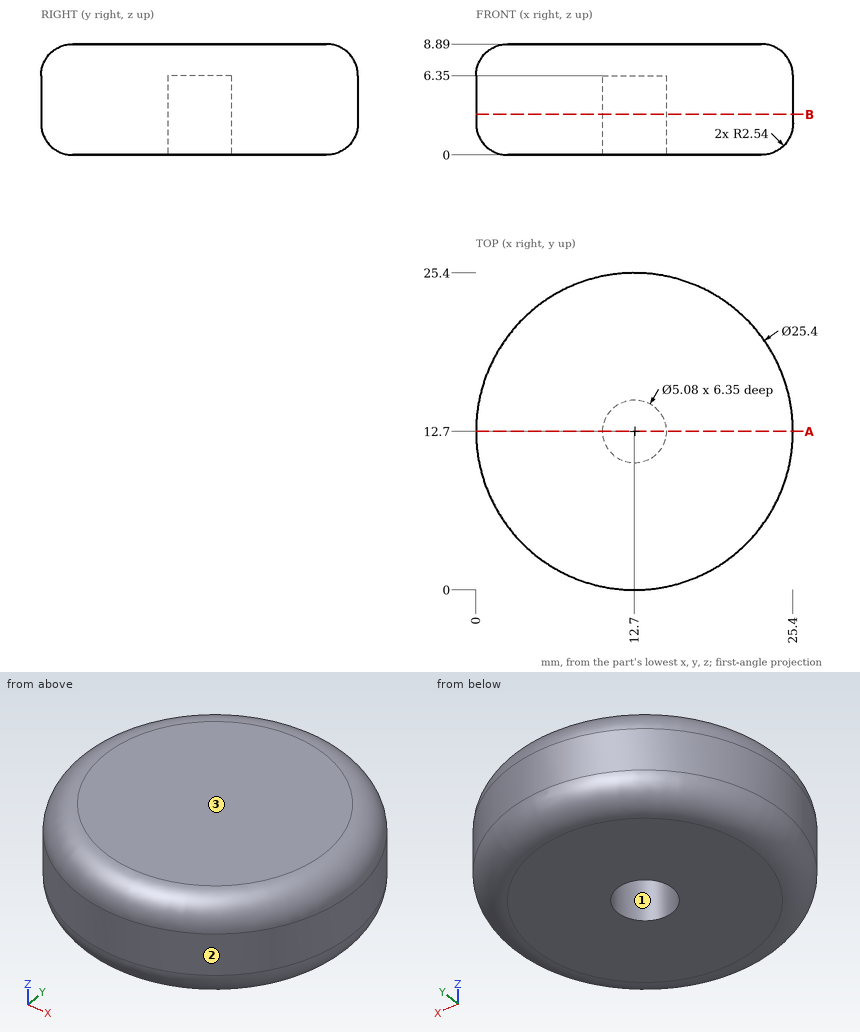
Could you check a few things on this drawing? It's one solid part, dimensions in mm from its lowest x, y, z. Coordinates: 2 decimals unless noted, no trailing zeros. Order: outer loops, then holes, each group sorted by start corner. A loop starts at its lowest first (then second) coordinate and runs counter-clockwise, first axis right, second up. Notation, with made-up numbers: M 75.5,-29 L 126.5,-29 A12 cw 126.5,-19 Z; hole C -31,-16.75 d7. An arc over 180 degrees is marked long. Answer as a JSON object with one key per item and string values. Group by question number.
(1) If we mould it in two halves opening along X, with no side actions, what happens to the marked faces 1, 2 and 3? For each: released by +X, released by -X, zero draft, split by the parting line, or undercut.
(2) I need wall thicknesses on probe 1 along Y at (x, z) = (12.7, 4); probe 2 along X at (y, z) = (14.75, 0.5); probe 3 along Y at (x, z) = (13.25, 1). Which ranges of each line are inside material? Lowest first, please.
(3) Suppose I cut it at B-B, the plane z = 3.25. Please give me the cut outline in (x, y).
(4) Suppose I cut it at A-A, the plane y = 12.7. Please give me the cut outline in (x, z).
(5) For pin 1 (3 mm diameter, centred on x = 10.5, z = 6.5, fed in from +Y); pin 2 (1 mm diameter, centred on y = 10, z = 4.5, fed in from -X); pin 3 (2.5 mm diameter, centred on x = 13, y = 12, fed in from -Z), each with a flat end and sliding along its axis, tell me the tip position at first contact or that it passes through.
Values found:
{
 "1": {"face 1": "undercut", "face 2": "split by the parting line", "face 3": "zero draft"},
 "2": {"probe 1": "y = 0 to 10.16, 15.24 to 25.4", "probe 2": "x = 1.21 to 11.2, 14.2 to 24.19", "probe 3": "y = 0.53 to 10.22, 15.18 to 24.87"},
 "3": {"outline": "C 12.7,12.7 d25.4; hole C 12.7,12.7 d5.08"},
 "4": {"outline": "M 0,2.54 A2.54 ccw 2.54,0 L 10.16,0 L 10.16,6.35 L 15.24,6.35 L 15.24,0 L 22.86,0 A2.54 ccw 25.4,2.54 L 25.4,6.35 A2.54 ccw 22.86,8.89 L 2.54,8.89 A2.54 ccw 0,6.35 Z"},
 "5": {"pin 1": "stops at y = 25.38", "pin 2": "stops at x = 0.19", "pin 3": "stops at z = 6.35"}
}
